Could you check a few things on this model? Use its own coordinates, in mm. Face numbers are marked on the shaded views. A direction names the side the tool comes from. Coordinates: 2 decimals unless noted, no trailing zeros. Write each loop counter-clockwise with the first axis right and the second up, starting at its lowest first coordinate (ties: lowest second). Pieces come first, ordered by that corner, then holes. Notation, with made-up numbers: M 87.5,46.25 L 97.5,46.25 A29 ccw 97.5,85.25 Z; hole C 53,-8.75 d8. An arc over 180 degrees is marked long. Write item = value, one per line.
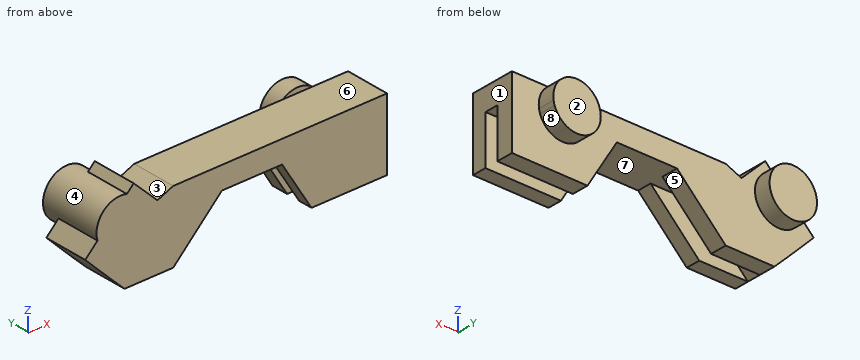
```python
from build123d import *

# Parameters (mm, degrees)
SKETCH2_R             = 4.25
BOSS_EXTRUDE1_DEPTH   = 6
BOSS_EXTRUDE1_2_DEPTH = 6
BOSS_EXTRUDE2_DEPTH   = 3
BOSS_EXTRUDE3_START   = -5
SKETCH2_9_R           = 4.25
BOSS_EXTRUDE3_DEPTH   = 5
BOSS_EXTRUDE4_DEPTH   = 2.56
SKETCH4_R             = 4.247751339
BOSS_EXTRUDE5_DEPTH   = 3


with BuildPart() as part:
    # Sketch2 → Boss-Extrude1 (new body)
    with BuildSketch(Plane(origin=(0, 0, 0), x_dir=(1, 0, 0), z_dir=(0, 1, 0))):
        with Locations(Location((-9.482754905, -1.788781285, 0), (0, 0, 270))):
            Circle(SKETCH2_R)
    extrude(amount=BOSS_EXTRUDE1_DEPTH)



with BuildPart() as body_2:
    # Sketch2 → Boss-Extrude1 2 (new body)
    with BuildSketch(Plane(origin=(0, 0, 0), x_dir=(1, 0, 0), z_dir=(0, 1, 0))):
        with BuildLine():
            Line((33.43268592, 0), (25.037974223, 0))
            ThreePointArc((25.037974223, 0), (29.235330072, 3.583138785), (33.43268592, 0))
        make_face()
    extrude(amount=BOSS_EXTRUDE1_2_DEPTH)


with BuildPart() as part_1:
    add(part.part)

    add(body_2.part)  # Boss-Extrude2 merges body 2
    # Sketch2_7 → Boss-Extrude2 (add)
    with BuildSketch(Plane(origin=(0, 0, 0), x_dir=(1, 0, 0), z_dir=(0, 1, 0))):
        with BuildLine():
            Line((0, 8.718626612), (-8.718626612, 8.718626612))
            Line((-8.718626612, 8.718626612), (-11.561455819, 5.875797405))
            Line((-11.561455819, 5.875797405), (-15.748205688, 1.58521084))
            Line((-15.748205688, 1.58521084), (-13.563084148, -0.5999107))
            ThreePointArc((-13.563084148, -0.5999107), (-6.477551085, 1.216422535), (-8.29388432, -5.869110529))
            Line((-8.29388432, -5.869110529), (-7.081497424, -7.081497424))
            Line((-7.081497424, -7.081497424), (-2.828427125, -2.828427125))
            Line((-2.828427125, -2.828427125), (0, -4))
            Line((0, -4), (38.28, -4))
            Line((38.28, -4), (38.28, 8.718626612))
            Line((38.28, 8.718626612), (24.755242586, 8.718626612))
            Line((24.755242586, 8.718626612), (19.499755178, 0))
            Line((19.499755178, 0), (8.718626612, 0))
            Line((8.718626612, 0), (0, 8.718626612))
        make_face()
        with BuildLine():
            Line((33.43268592, 0), (25.037974223, 0))
            ThreePointArc((25.037974223, 0), (29.235330072, 3.583138785), (33.43268592, 0))
        make_face(mode=Mode.SUBTRACT)
    extrude(amount=BOSS_EXTRUDE2_DEPTH)

    # Sketch2_9 → Boss-Extrude3 (add)
    with BuildSketch(Plane(origin=(0, 0, 0), x_dir=(1, 0, 0), z_dir=(0, 1, 0)).offset(BOSS_EXTRUDE3_START)):
        with BuildLine():
            Line((8.718626612, 0), (0, 0))
            Line((0, 0), (-8.718626612, 8.718626612))
            Line((-8.718626612, 8.718626612), (-11.561455819, 5.875797405))
            Line((-11.561455819, 5.875797405), (-15.748205688, 1.58521084))
            Line((-15.748205688, 1.58521084), (-13.563084148, -0.5999107))
            ThreePointArc((-13.563084148, -0.5999107), (-8.882296448, 2.418587208), (-5.232754905, -1.788781285))
            ThreePointArc((-5.232754905, -1.788781285), (-6.083107866, -4.339251832), (-8.29388432, -5.869110529))
            Line((-8.29388432, -5.869110529), (-7.081497424, -7.081497424))
            Line((-7.081497424, -7.081497424), (-2.828427125, -2.828427125))
            Line((-2.828427125, -2.828427125), (0, -4))
            Line((0, -4), (26.598535457, -4))
            Line((26.598535457, -4), (31.872124686, -4))
            Line((31.872124686, -4), (38.28, -4))
            Line((38.28, -4), (38.28, 0))
            Line((38.28, 0), (34.190660144, 0))
            Line((34.190660144, 0), (33.43268592, 0))
            Line((33.43268592, 0), (25.037974223, 0))
            Line((25.037974223, 0), (24.28, 0))
            Line((24.28, 0), (19.499755178, 0))
            Line((19.499755178, 0), (8.718626612, 0))
        make_face()
        with Locations(Location((-9.482754905, -1.788781285, 0), (0, 0, 163.75565512))):
            Circle(SKETCH2_9_R)
    extrude(amount=BOSS_EXTRUDE3_DEPTH)

    # Sketch3 → Boss-Extrude4 (add)
    with BuildSketch(Plane(origin=(0, -5, 0), x_dir=(-1, 0, 0), z_dir=(0, -1, 0))):
        Polygon((-38.28, -4), (-38.28, 8.718626612), (-24.755242586, 8.718626612), (-19.499755178, 0), (-8.718626612, 0), (0, 8.718626612), (8.718626612, 8.718626612), (15.748205688, 1.58521084), (13.563084148, -0.5999107), (7.081497424, -7.081497424), (2.828427125, -2.828427125), (0, -4), align=None)
    extrude(amount=-BOSS_EXTRUDE4_DEPTH)

    # Sketch4 → Boss-Extrude5 (add)
    with BuildSketch(Plane(origin=(0, 3, 0), x_dir=(1, 0, 0), z_dir=(0, 1, 0))):
        with Locations((29.235330072, -0.66)):
            Circle(SKETCH4_R)
    extrude(amount=BOSS_EXTRUDE5_DEPTH)


solid = part_1.part
```
Item 1: Imagine slicing it at B-B (z = -7.5). Write out the boundary of the cut face in (x, y).
Numbers:
outline = M -9.94,-5 L 1.22,-5 L 1.22,-2.44 L -7.5,-2.44 L -7.5,0 L 1.22,0 L 1.22,3 L -9.94,3 Z; M 24.02,-5 L 38.28,-5 L 38.28,-2.44 L 24.02,-2.44 Z; M 24.02,0 L 38.28,0 L 38.28,3 L 24.02,3 Z
Item 2: For the marked faces 4, 5, 6, 7 and 8, which set-ups out of +Z, -Z, +X, -X, +Y, -Y let a thin tool reach every point of the face, with its end or its side?
Numbers:
face_4 = +Y
face_5 = -Z, +Y, -Y
face_6 = +Z, +X, -Y
face_7 = -Z
face_8 = -Z, +Y
Item 3: Imagine slicing it at C-C (x = 20.5). Write out the boundary of the cut face in (y, z).
Numbers:
outline = M -5,-1.66 L -2.44,-1.66 L -2.44,0 L 0,0 L 0,-1.66 L 3,-1.66 L 3,4 L -5,4 Z
Item 4: I'm going to push a flat-ended pin straight in: P1, Ø3, axis at x = 24, y = -3.5, coming from the +Z side. Where does the tip first touch, or does it pass through?
Numbers:
P1 = 4
Item 5: If we mould it in two halves opening along X, with no side actions, what happens to the marked faces 1, 2 and 3? For each: pulls with the +X half, pulls with the -X half, needs draft (parallel to the pull), parting line crosses it, or undercut.
Numbers:
face_1 = pulls with the +X half
face_2 = needs draft
face_3 = undercut
Item 6: Imagine slicing it at D-D (x = 8). Write out the boundary of the cut face in (y, z), and give its area (3 significant figures).
Numbers:
outline = M -5,-0.72 L -2.44,-0.72 L -2.44,0 L 0,0 L 0,-0.72 L 3,-0.72 L 3,4 L -5,4 Z
area = 36.0 mm²
Item 7: If I drill on line 1 along Y through (x, z) = (7.5, -1); line 2 along Y through (x, z) = (4, 3); line 3 along X through (y, z) = (1.5, -6.75), over which ranges is the centre line in solid material (lowest first)?
Numbers:
line_1 = -5 to -2.44, 0 to 3
line_2 = -5 to 3
line_3 = -10.69 to 1.97, 23.57 to 38.28
